```python
from build123d import *

# Parameters (mm, degrees)
F0_R     = 13.335
F0_R_2   = 9.525
F1_DEPTH = 1117.6
F3_D     = 3.175
F3_DEPTH = 25.4
F3_TIP   = 0.9538662327
F4_D     = 3.175
F4_DEPTH = 25.4
F4_TIP   = 0.9538662327
F5_D     = 3.175
F5_DEPTH = 25.4
F5_TIP   = 0.9538662327
F6_D     = 3.175
F6_DEPTH = 25.4
F6_TIP   = 0.9538662327


with BuildPart() as f1:
    # F0 (on Right) → F1 (new body)
    with BuildSketch(Plane.YZ):
        Circle(F0_R)
        Circle(F0_R_2, mode=Mode.SUBTRACT)
    extrude(amount=F1_DEPTH)

    # F3 (one way)
    with BuildSketch(Plane.XY):
        with Locations((17.9905965924, 0)):
            Circle(F3_D / 2)
    extrude(amount=-F3_DEPTH, mode=Mode.SUBTRACT)
    with Locations(Plane.XY):
        with Locations((17.9905965924, 0)):
            with Locations((0, 0, -(F3_DEPTH + F3_TIP / 2))):  # 118° drill point
                Cone(0, F3_D / 2, F3_TIP, mode=Mode.SUBTRACT)

    # F4 (one way)
    with BuildSketch(Plane.XY):
        with Locations((36.9387045503, 0)):
            Circle(F4_D / 2)
    extrude(amount=-F4_DEPTH, mode=Mode.SUBTRACT)
    with Locations(Plane.XY):
        with Locations((36.9387045503, 0)):
            with Locations((0, 0, -(F4_DEPTH + F4_TIP / 2))):  # 118° drill point
                Cone(0, F4_D / 2, F4_TIP, mode=Mode.SUBTRACT)

    # F5 (one way)
    with BuildSketch(Plane.XY):
        with Locations((76.2924551964, 0)):
            Circle(F5_D / 2)
    extrude(amount=-F5_DEPTH, mode=Mode.SUBTRACT)
    with Locations(Plane.XY):
        with Locations((76.2924551964, 0)):
            with Locations((0, 0, -(F5_DEPTH + F5_TIP / 2))):  # 118° drill point
                Cone(0, F5_D / 2, F5_TIP, mode=Mode.SUBTRACT)

    # F6 (one way)
    with BuildSketch(Plane.XY):
        with Locations((57.1621619165, 0)):
            Circle(F6_D / 2)
    extrude(amount=-F6_DEPTH, mode=Mode.SUBTRACT)
    with Locations(Plane.XY):
        with Locations((57.1621619165, 0)):
            with Locations((0, 0, -(F6_DEPTH + F6_TIP / 2))):  # 118° drill point
                Cone(0, F6_D / 2, F6_TIP, mode=Mode.SUBTRACT)


solid = f1.part
```
Check sheet for the modelled part. Datum: model origin and axes. Units: mm. Coordinates: 2 decimals unless noted, no trailing zeros. Write each loop counter-clockwise with the first axis right and the second up, starting at its lowest first coordinate (ties: lowest second). Pieces come first, ordered by that corner, then holes. Notation, with made-up numbers: (-28, 59) -> (-7, 59) arc R21 ccw to (-7, 67) -> close; hole circle Ø5 at (-18.5, 21.5). An arc over 180 degrees is marked (long way). Use a Markdown table: item, result.
1. Sectioned sample at A-A (z = 0). Enter the section's corners in (x, y) (3 decimals), plus the area to 3 significant figures.
Reported:
| item | result |
|---|---|
| outline | (0, -13.335) -> (1117.6, -13.335) -> (1117.6, -9.525) -> (0, -9.525) -> close; (0, 9.525) -> (1117.6, 9.525) -> (1117.6, 13.335) -> (0, 13.335) -> close |
| area | 8,520 mm2 |
2. Release check for a two-part mould opening along Z. For faces 1 (the cylindrical face through (550.98, -1.74, 13.22)), 2 (the cylindrical face through (550.977, -7.559, -5.796)), 3 (the flat face through (0, 9, -6)) record: pulls with the +Z half, pulls with the -Z half, needs draft (parallel to the pull), parting line crosses it, or undercut.
Reported:
| item | result |
|---|---|
| face 1 | parting line crosses it |
| face 2 | undercut |
| face 3 | needs draft |
3. Scan lines: line 1 along X through (y, z) = (0, -11.7); line 2 along Y through (x, z) = (102, -1); line 3 along Z through (x, y) = (459, 0) (3 decimals). Record each from-to range of solid material in increasing order.
Reported:
| item | result |
|---|---|
| line 1 | x = 0 to 16.4, 19.58 to 35.35, 38.53 to 55.57, 58.75 to 74.7, 77.88 to 1117.6 |
| line 2 | y = -13.3 to -9.47, 9.47 to 13.3 |
| line 3 | z = -13.335 to -9.525, 9.525 to 13.335 |
4. Sectioned sample at B-B (x = 315). Enter the section's corners in (y, z) (3 decimals), plus the area to 3 significant figures.
Reported:
| item | result |
|---|---|
| outline | circle Ø26.67 at (0, 0); hole circle Ø19.05 at (0, 0) |
| area | 274 mm2 |
5. Go/stop test with flat-tipped pins: pin 1 Ø5 at (x, y) = (724.5, -4) entering from +Z; pin 2 Ø1.9 at (x, y) = (36.94, 0) entering from -Z; pin 3 Ø12 at (x, y) = (641, -9.5) entering from +Z; pin 4 Ø4 at (y, z) = (1, -7) entering from +X. Record where each tip stops, or that it passes through.
Reported:
| item | result |
|---|---|
| pin 1 | stops at z = 13.25 |
| pin 2 | stops at z = 9.48 |
| pin 3 | stops at z = 12.87 |
| pin 4 | passes through |
